Can you work these out from the model? Positions are in its coordinate system, mm. Face numbers are marked on the shaded views. Coordinates: 2 decimals unless noted, no trailing zeros. Order: outer loops, then holes, each group sorted by start corner. A loop starts at its lowest first (then second) coordinate and runs counter-clockwise, first axis right, second up. Notation, with made-up numbers: (21.25, 13.25) -> (50.25, 13.25) arc R5 ccw to (50.25, 17.25) -> close; hole circle Ø11 at (69.5, 5). An arc over 180 degrees is marked (long way). Return JSON: item names as keys, results as strings. Group by question number.
1) For pin 1 (4 mm diameter, centred on x = 6, z = 6, fed in from -Y); pin 2 (3 mm diameter, centred on y = 20, z = -14, fed in from +X); pin 3 (3 mm diameter, centred on x = 6.5, y = 41, fed in from +Z); pin 4 (8 mm diameter, centred on y = 45, z = 19.5, fed in from -X), each with a flat end and sliding along its axis, tell me the tip position at first contact or that it passes through.
2) If we section it at A-A, the plane x = 0: Please give me the cut outline in (y, z), then the cut area to 3 significant figures.
3) If I drill on probe 1 along Z at (x, y) = (0, 52.5); probe 2 along X at (y, z) = (57, 0); probe 3 along Y at (x, z) = (-37.5, 16), over which ranges is the centre line in solid material (lowest first)? Write a range as from..to.
4) If we section it at C-C, the plane y = 31: Please give me the cut outline in (x, z), then the cut area to 3 significant figures.
5) If we section it at B-B, the plane z = 0: Please give me the cut outline in (x, y).
6) Thinking about a two-plate mould opening in X: for the marked faces 1, 2 and 3, which applies, +X half, -X half, draft (parallel to the pull), parting line (faces both ways), or undercut?
from build123d import *
from build123d import SkipClean  # not in build123d's __all__

# Parameters (mm, degrees)
F2_DEPTH = 2
F1_W     = 2
F1_H     = 9
F6_DEPTH = 3


with BuildPart() as f2:
    # F0 (on Front) → F2 (new body)
    with BuildSketch(Plane.XZ):
        Polygon((-52.5, -46), (52.5, -46), (46.5, 34), (30, 46), (-30, 46), (-46.5, 34), align=None)
    extrude(amount=-F2_DEPTH)

    # F1 (on Top) → F3 (revolve, cut)
    with BuildSketch(Plane.XY):
        Polygon((-20, 0), (0, 0), (0, 50), (-7.2, 50), (-40, 0), (-22, 0), align=None)
    revolve(axis=Axis((0, 25, 0), (0, 1, 0)), mode=Mode.SUBTRACT)

    # F1 (on Top) → F4 (revolve)
    with BuildSketch(Plane.XY):
        Polygon((-40, 0), (-7.2, 50), (-9.2, 50), (-42, 0), align=None)
        with Locations((-8.2, 54.5)):
            Rectangle(F1_W, F1_H)
    with SkipClean():  # cleaning this boolean's faces spoils the solid; the shape is the same uncleaned
        revolve(axis=Axis((0, 2, 0), (0, -1, 0)))

    # F5 (on face) → F6 (join)
    with BuildSketch(Plane(origin=(0, 59, 0), x_dir=(-1, 0, 0), z_dir=(0, 1, 0))):
        with BuildLine():
            Line((-6.2, -3.6606010435), (-6.2, 0))
            Line((-6.2, 0), (-6.2, 3.6606010435))
            ThreePointArc((-6.2, 3.6606010435), (-7.2, 0), (-6.2, -3.6606010435))
        make_face()
        with BuildLine():
            ThreePointArc((7.2, 0), (6.9455021417, 1.8973665961), (6.2, 3.6606010435))
            Line((6.2, 3.6606010435), (6.2, -3.6606010435))
            ThreePointArc((6.2, -3.6606010435), (6.9455021417, -1.8973665961), (7.2, 0))
        make_face()
    with SkipClean():  # cleaning this boolean's faces spoils the solid; the shape is the same uncleaned
        extrude(amount=-F6_DEPTH)


solid = f2.part
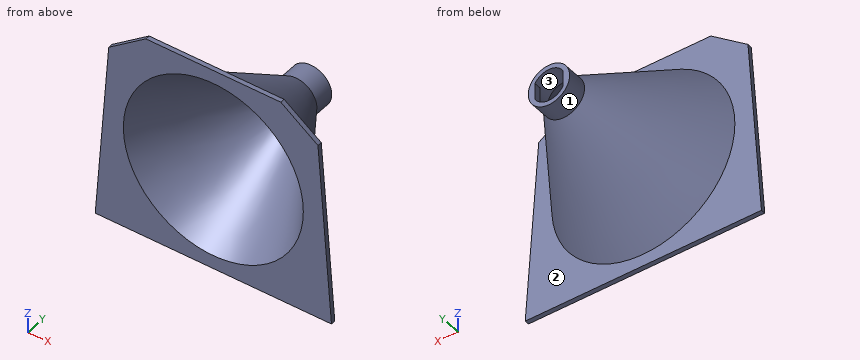
Result sheet:
{
 "1": {"pin 1": "stops at y = 44.99", "pin 2": "stops at x = 26.62", "pin 3": "stops at z = 14.88", "pin 4": "passes through"},
 "2": {"outline": "(0, -46) -> (2, -46) -> (2, -40.69) -> (50, -9.2) -> (59, -9.2) -> (59, -7.2) -> (50, -7.2) -> (0, -40) -> close; (0, 40) -> (50, 7.2) -> (59, 7.2) -> (59, 9.2) -> (50, 9.2) -> (2, 40.69) -> (2, 46) -> (0, 46) -> close", "area": "255 mm2"},
 "3": {"probe 1": "z = -9.2..-7.2, 7.2..9.2", "probe 2": "x = -9.2..-6.2, 6.2..9.2", "probe 3": "y = 0..2"},
 "4": {"outline": "circle Ø43.33 at (0, 0); hole circle Ø39.33 at (0, 0)", "area": "260 mm2"},
 "5": {"outline": "(-49.05, 0) -> (-40, 0) -> (-7.2, 50) -> (-7.2, 56) -> (-6.2, 56) -> (-6.2, 59) -> (-9.2, 59) -> (-9.2, 50) -> (-40.69, 2) -> (-49.05, 2) -> close; (6.2, 56) -> (7.2, 56) -> (7.2, 50) -> (40, 0) -> (49.05, 0) -> (49.05, 2) -> (40.69, 2) -> (9.2, 50) -> (9.2, 59) -> (6.2, 59) -> close"},
 "6": {"face 1": "parting line", "face 2": "draft", "face 3": "undercut"}
}
